Answer from the drawing. Dimensions are ordinates in mm from the lowest x, y and z of the part. A direction names the side the tool comes from. Coordinates: 2 decimals unless noted, no trailing zeros. Loops run counter-clockwise (first coordinate to the right, second up) from the corner with the lowest first, then second, coordinate; pieces in that order, holes last. Notation, with made-up numbers: (18.5, 60) - (74.5, 60) arc R12 cw to (74.5, 83) - close; hole circle Ø5 at (-0.75, 27.5). An arc over 180 degrees is marked (long way). Use one line per item in the form item = value. Start each with the question number.
1) Consider line 1 (X direction, y = 8.25, z = 5.25) (3 decimals); line 2 (Z direction, x = 76.25, y = 11); line 3 (Z direction, x = 76.25, y = 3.75) (3 decimals). Determine where each line is inside the solid, lowest interval first.
2) The mould has two halves that part along X. Classify the marked faces 1, 2, 3 and 4: released by +X, released by -X, zero draft, split by the parting line, or undercut.
3) Which of the six approach directions +Z, -Z, +X, -X, +Y, -Y give full straight-line access (tool end or side, diameter ignored) to the marked faces 5 and 6?
4) A cutting plane is placed at D-D (x = 55.5). Give the vertices of the cut face in (y, z).
5) Each of these flat-tipped pins is pushed along its axis until it touches: P1, Ø3.5, axis at x = 76.25, z = 55.75, coming from the -Y side; P2, Ø1.6, axis at x = 75.5, z = 55, coming from the +Y side; P3, Ø1.2, axis at x = 63, z = 60.5, coming from the -Y side. Where does it stop, or does it pass through?
6) A cutting plane is placed at A-A (y = 4.75). Give the vertices of the cut face in (x, z) (3 decimals).
7) A cutting plane is placed at C-C (z = 5.25). Give the vertices of the cut face in (x, y) (3 decimals).
8) A cutting plane is placed at B-B (x = 76.25). State how many separate pieces and enclosed holes the cut face has, and give its area (3 significant figures).
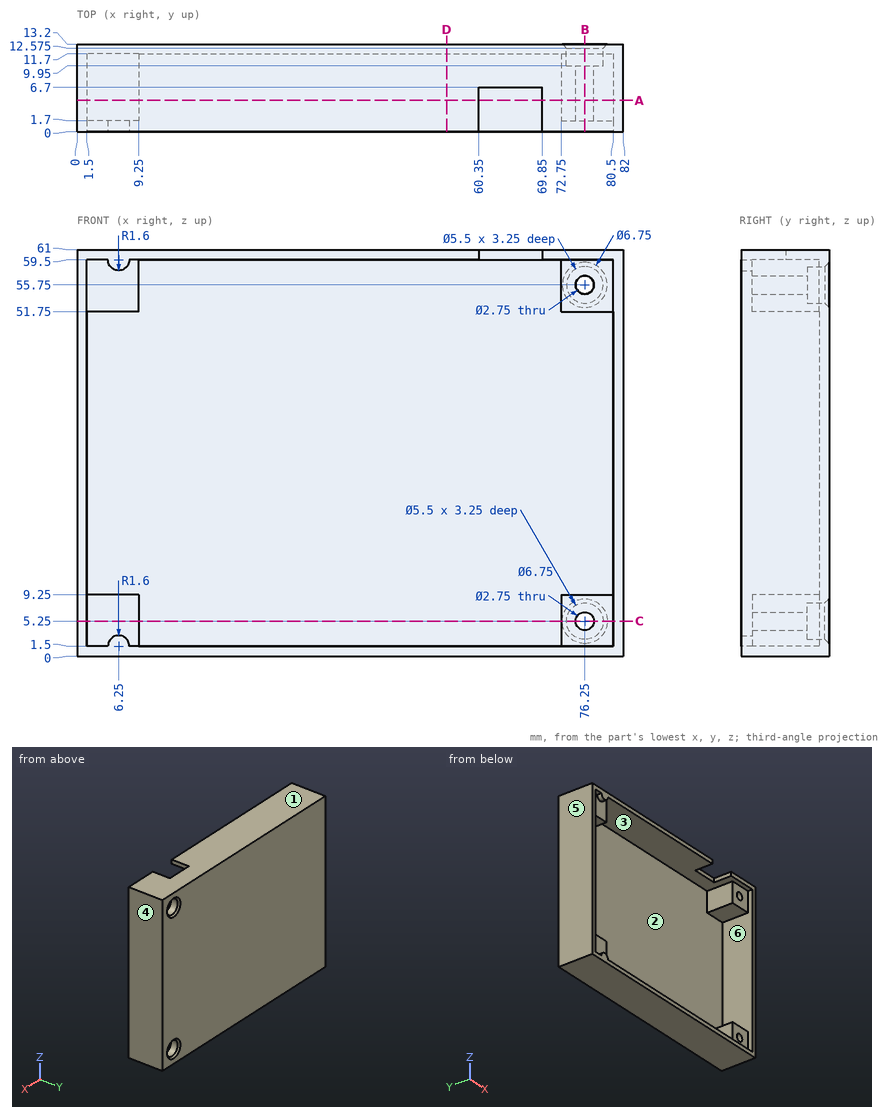
Found:
q1.line_1 = 0 to 9.25, 72.75 to 74.875, 77.625 to 82
q1.line_2 = 0 to 2.5, 8 to 9.25, 51.75 to 53, 58.5 to 61
q1.line_3 = 0 to 3.875, 6.625 to 9.25, 51.75 to 54.375, 57.125 to 61
q2.face_1 = zero draft
q2.face_2 = undercut
q2.face_3 = undercut
q2.face_4 = released by +X
q3.face_5 = +Z, -Z, -X, +Y, -Y
q3.face_6 = -Y
q4.outline = (0, 0) - (13.2, 0) - (13.2, 61) - (0, 61) - (0, 59.5) - (11.7, 59.5) - (11.7, 1.5) - (0, 1.5) - close
q5.P1 = 1.7
q5.P2 = 9.95
q5.P3 = 6.7
q6.outline = (0, 0) - (82, 0) - (82, 61) - (69.85, 61) - (69.85, 59.5) - (72.75, 59.5) - (72.75, 51.75) - (80.5, 51.75) - (80.5, 9.25) - (72.75, 9.25) - (72.75, 1.5) - (9.25, 1.5) - (9.25, 9.25) - (1.5, 9.25) - (1.5, 51.75) - (9.25, 51.75) - (9.25, 59.5) - (60.35, 59.5) - (60.35, 61) - (0, 61) - close; hole circle Ø2.75 at (76.25, 5.25); hole circle Ø2.75 at (76.25, 55.75)
q7.outline = (0, 0) - (1.5, 0) - (1.5, 1.7) - (9.25, 1.7) - (9.25, 11.7) - (72.75, 11.7) - (72.75, 1.7) - (74.875, 1.7) - (74.875, 9.95) - (73.5, 9.95) - (73.5, 12.575) - (72.875, 13.2) - (0, 13.2) - close; (77.625, 1.7) - (80.5, 1.7) - (80.5, 0) - (82, 0) - (82, 13.2) - (79.625, 13.2) - (79, 12.575) - (79, 9.95) - (77.625, 9.95) - close
q8.separate_pieces = 3
q8.enclosed_holes = 0
q8.area = 200 mm^2
